Here's the drawing with two shaded views (mm, measured from the low corner). I have some questions. A direction names the side the tool comes from. Round coordinates to 2 decimals unless told otherwise and drop trailing zeros. Order: outer loops, then holes, each group sorted by start corner. A loop starts at its lowest first (then second) coordinate and runs counter-clockwise, first axis right, second up. Notation, with made-up numbers: (-31, 88) -> (4, 88) arc R24 ccw to (4, 111) -> close; hole circle Ø3 at (45, 12.25). An arc over 180 degrees is marked (long way). Answer in a Markdown table with one row per item.
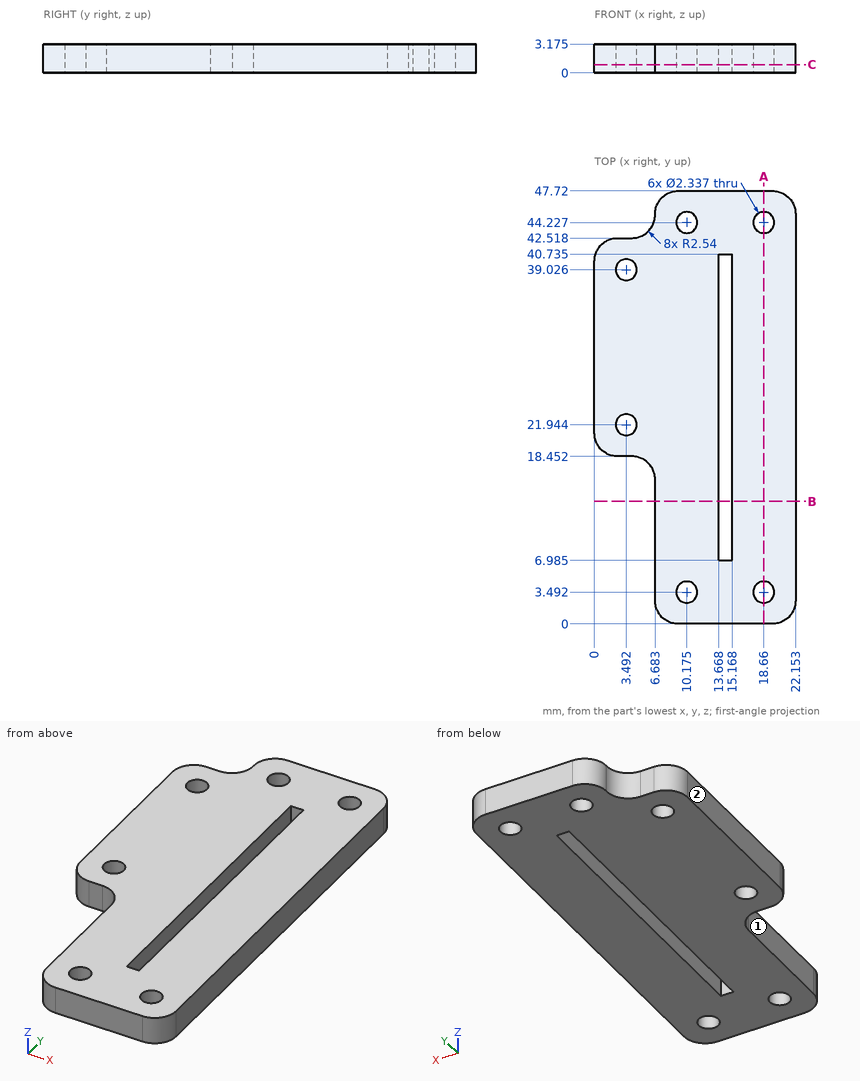
1. Please list where these lines run through material, in increasing order: line 1 along Y through (x, z) = (3.5, 1.6) (1 decimal); line 2 along Y through (x, z) = (18.66, 1.45) (1 decimal); line 3 along X through (y, z) = (14.5, 0.4).
Numbers:
| item | result |
|---|---|
| line 1 | y = 18.5 to 20.8, 23.1 to 37.9, 40.2 to 42.5 |
| line 2 | y = 0 to 2.3, 4.7 to 43.1, 45.4 to 47.7 |
| line 3 | x = 6.68 to 13.67, 15.17 to 22.15 |
2. For the marked faces 1 and 2, which set-ups out of +Z, -Z, +X, -X, +Y, -Y let a thin tool reach every point of the face, with its end or its side?
Numbers:
| item | result |
|---|---|
| face 1 | +Z, -Z, -X, -Y |
| face 2 | +Z, -Z, -X, +Y, -Y |
3. Suppose I cut it at B-B on y = 13.5. Write out the boundary of the cut face in (x, z) (1 decimal).
Numbers:
| item | result |
|---|---|
| outline | (6.7, 0) -> (13.7, 0) -> (13.7, 3.2) -> (6.7, 3.2) -> close; (15.2, 0) -> (22.2, 0) -> (22.2, 3.2) -> (15.2, 3.2) -> close |
4. Suppose I cut it at A-A on x = 18.66. Write out the boundary of the cut face in (y, z) (1 decimal).
Numbers:
| item | result |
|---|---|
| outline | (0, 0) -> (2.3, 0) -> (2.3, 3.2) -> (0, 3.2) -> close; (4.7, 0) -> (43.1, 0) -> (43.1, 3.2) -> (4.7, 3.2) -> close; (45.4, 0) -> (47.7, 0) -> (47.7, 3.2) -> (45.4, 3.2) -> close |
5. Suppose I cut it at C-C on z = 0.9. State how many separate pieces and enclosed holes the cut face has, then the cut area to 3 significant figures.
Numbers:
| item | result |
|---|---|
| separate pieces | 1 |
| enclosed holes | 7 |
| area | 817 mm2 |
6. For pin 1 Ø5 at (x, y) = (18, 38.5) entering from -Z; pin 2 Ø1.9 at (x, y) = (10.18, 44.23) entering from +Z; pin 3 Ø1.3 at (x, z) = (3, 2.5) entering from -Y; pin 4 Ø1.3 at (x, z) = (3.5, 2.5) entering from +Y, each with a flat end and sliding along its axis, tell me the tip position at first contact or that it passes through.
Numbers:
| item | result |
|---|---|
| pin 1 | stops at z = 0 |
| pin 2 | passes through |
| pin 3 | stops at y = 18.45 |
| pin 4 | stops at y = 42.52 |
